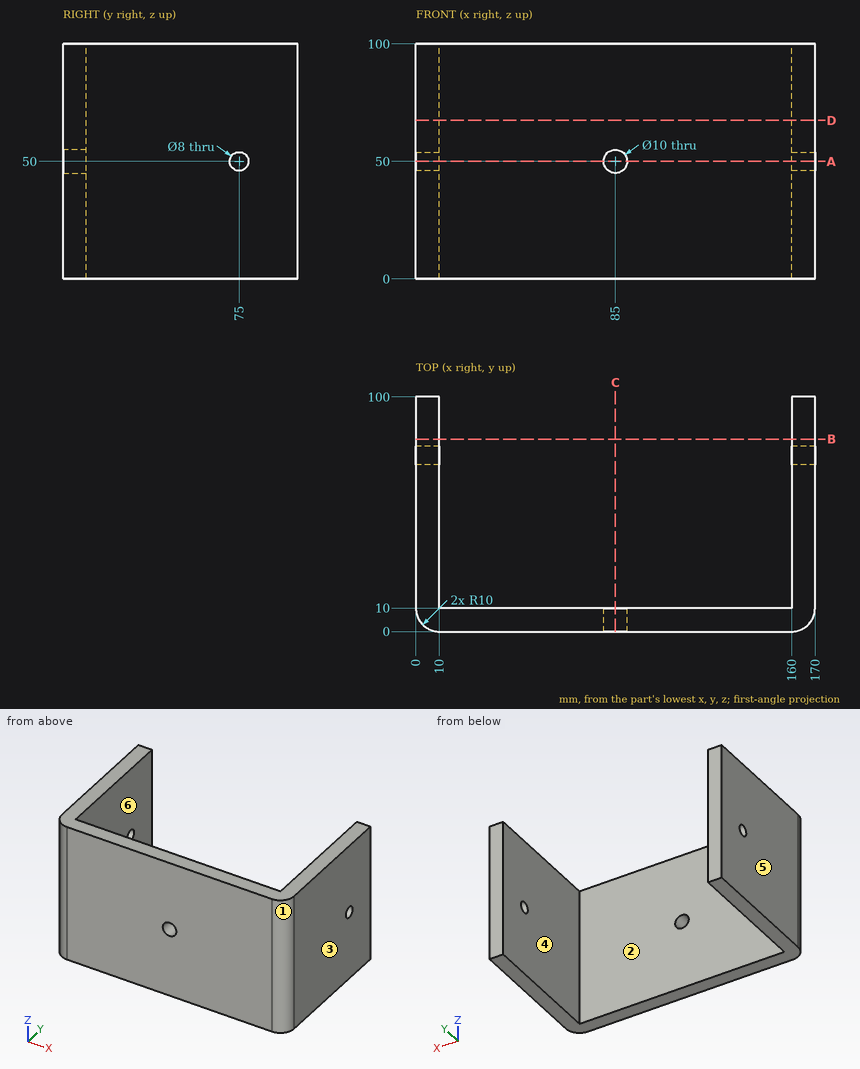
The drawing under review shows one solid part. Ordinate dimensions are in mm from its lowest x, y, z. A direction names the side the tool comes from. Coordinates: 2 decimals unless noted, no trailing zeros. Order: outer loops, then holes, each group sorted by start corner. A loop starts at its lowest first (then second) coordinate and runs counter-clockwise, first axis right, second up. Notation, with made-up numbers: (-37, -28.75) -> (-25, -28.75) arc R11 ccw to (-25, -24.75) -> close; hole circle Ø2 at (34, 11.5). An arc over 180 degrees is marked (long way). Answer in a Markdown table with one row per item.
(1) Insertion check: pin 1 (10 mm diameter, centred on x = 97.5, z = 79, fed in from +Y); pin 2 (6 mm diameter, centred on x = 139, y = 15.5, fed in from -Z). Each pin has a flat end and moves straight along its axis. Give the tip position at first contact, or say it passes through.
Answers:
| item | result |
|---|---|
| pin 1 | y = 10 |
| pin 2 | through |
(2) Consider section D-D (z = 67.5). Write out the cut boundary in (x, y).
Answers:
| item | result |
|---|---|
| outline | (0, 10) arc R10 ccw to (10, 0) -> (160, 0) arc R10 ccw to (170, 10) -> (170, 100) -> (160, 100) -> (160, 10) -> (10, 10) -> (10, 100) -> (0, 100) -> close |
(3) Consider section B-B (y = 82). Write out the cut boundary in (x, z), plus the area to 3 significant figures.
Answers:
| item | result |
|---|---|
| outline | (0, 0) -> (10, 0) -> (10, 100) -> (0, 100) -> close; (160, 0) -> (170, 0) -> (170, 100) -> (160, 100) -> close |
| area | 2,000 mm² |
(4) Consider section C-C (x = 85). Write out the cut boundary in (y, z), plus the area to 3 significant figures.
Answers:
| item | result |
|---|---|
| outline | (0, 0) -> (10, 0) -> (10, 45) -> (0, 45) -> close; (0, 55) -> (10, 55) -> (10, 100) -> (0, 100) -> close |
| area | 900 mm² |
(5) Wall thickness on line 1 along X through (y, z) = (75, 15.5); line 2 along Y through (x, z) = (93.5, 94.5); line 3 along Y through (x, z) = (163, 50): over which ranges is each line inside the solid? List them lowest first.
Answers:
| item | result |
|---|---|
| line 1 | 0 to 10, 160 to 170 |
| line 2 | 0 to 10 |
| line 3 | 0.46 to 71, 79 to 100 |
(6) The part is to be moulded in two halves that separate along X. For the marked faces 3, 4, 5 and 6, say which applies: +X half, -X half, draft (parallel to the pull), parting line (faces both ways), or undercut.
Answers:
| item | result |
|---|---|
| face 3 | +X half |
| face 4 | undercut |
| face 5 | -X half |
| face 6 | undercut |
(7) Machinability: for the marked faces 1 and 2, which of the approach directions +Z, -Z, +X, -X, +Y, -Y give a long, thin tool a straight path to every point of the face, cutting with its end or side? Answer none if there is none.
Answers:
| item | result |
|---|---|
| face 1 | +Z, -Z, +X, -Y |
| face 2 | +Z, -Z, +Y |
(8) Consider section A-A (z = 50). Write out the cut boundary in (x, y).
Answers:
| item | result |
|---|---|
| outline | (0, 10) arc R10 ccw to (10, 0) -> (80, 0) -> (80, 10) -> (10, 10) -> (10, 71) -> (0, 71) -> close; (0, 79) -> (10, 79) -> (10, 100) -> (0, 100) -> close; (90, 0) -> (160, 0) arc R10 ccw to (170, 10) -> (170, 71) -> (160, 71) -> (160, 10) -> (90, 10) -> close; (160, 79) -> (170, 79) -> (170, 100) -> (160, 100) -> close |
